Model file for the job. Use its own axes, mm. Face numbers are marked on the shaded views. A direction names the side the tool comes from. Round coordinates to 2 decimals unless told otherwise and drop trailing zeros. Order: outer loops, then holes, each group sorted by start corner. A loop starts at its lowest first (then second) coordinate and runs counter-clockwise, first axis right, second up. Notation, with made-up numbers: (40.25, 46) - (70.25, 46) arc R4 ccw to (70.25, 52) - close; hole circle Ø4 at (-9.5, 58.25). An arc over 180 degrees is marked (long way). Use one line per item in the form item = value.
from build123d import *

# Parameters (mm, degrees)
SKETCH1_W           = 40
SKETCH1_H           = 20
BOSS_EXTRUDE1_DEPTH = 10
SKETCH2_R           = 5.15
CUT_EXTRUDE1_DEPTH  = 2.4
CUT_EXTRUDE2_DEPTH  = 31
FILLET1_R           = 2
SKETCH4_W           = 0.5
SKETCH4_H           = 10
CUT_EXTRUDE3_DEPTH  = 0.5
SKETCH5_W           = 0.5
SKETCH5_H           = 20
CUT_EXTRUDE4_DEPTH  = 0.5
SKETCH6_W           = 0.5
SKETCH6_H           = 10
CUT_EXTRUDE5_DEPTH  = 0.5
FILLET2_R           = 1
SKETCH8_W           = 14.3
SKETCH8_H           = 7
CUT_EXTRUDE7_DEPTH  = 3.3
SKETCH9_R           = 1.6
CUT_EXTRUDE8_DEPTH  = 10
CUT_EXTRUDE9_DEPTH  = 1.25
FILLET4_R           = 0.5


# Some blends are built 0.0001 mm under size
with BuildPart() as part:
    # Sketch1 → Boss-Extrude1 (new body)
    with BuildSketch(Plane(origin=(0, 0, 0), x_dir=(1, 0, 0), z_dir=(0, 1, 0))):
        Rectangle(SKETCH1_W, SKETCH1_H)
    extrude(amount=BOSS_EXTRUDE1_DEPTH)

    # Sketch2 → Cut-Extrude1 (cut)
    with BuildSketch(Plane.XZ):
        with Locations(Location((0, 0, 0), (0, 0, 270))):
            Circle(SKETCH2_R)
        with Locations(Location((12, 0, 0), (0, 0, 270))):
            Circle(SKETCH2_R)
        with Locations(Location((-12, 0, 0), (0, 0, 270))):
            Circle(SKETCH2_R)
    extrude(amount=-CUT_EXTRUDE1_DEPTH, mode=Mode.SUBTRACT)

    # Sketch3 → Cut-Extrude2 (cut, through all)
    with BuildSketch(Plane.XY.offset(10)):
        Polygon((18, 10), (14.75, 6.75), (14.75, 5.25), (13.25, 5.25), (13.25, 6.75), (10, 10), align=None)
    extrude(amount=-CUT_EXTRUDE2_DEPTH, mode=Mode.SUBTRACT)

    # Fillet1
    fillet1_edges = [part.edges().sort_by_distance(p)[0] for p in [
        (20, 10, 0),
        (-20, 10, 0),
        (-20, 5, -10),
        (20, 5, -10),
        (20, 5, 10),
        (-20, 5, 10),
    ]]
    fillet(fillet1_edges, radius=FILLET1_R - 0.0001)  # a hair under: the kernel refuses the full size

    # Sketch4 → Cut-Extrude3 (cut)
    with BuildSketch(Plane.XY.offset(10)):
        with Locations((0, 5)):
            Rectangle(SKETCH4_W, SKETCH4_H)
    extrude(amount=-CUT_EXTRUDE3_DEPTH, mode=Mode.SUBTRACT)

    # Sketch5 → Cut-Extrude4 (cut)
    with BuildSketch(Plane(origin=(0, 10, 0), x_dir=(1, 0, 0), z_dir=(0, 1, 0))):
        Rectangle(SKETCH5_W, SKETCH5_H)
    extrude(amount=-CUT_EXTRUDE4_DEPTH, mode=Mode.SUBTRACT)

    # Sketch6 → Cut-Extrude5 (cut)
    with BuildSketch(Plane(origin=(0, 0, -10), x_dir=(-1, 0, 0), z_dir=(0, 0, -1))):
        with Locations((0, 5)):
            Rectangle(SKETCH6_W, SKETCH6_H)
    extrude(amount=-CUT_EXTRUDE5_DEPTH, mode=Mode.SUBTRACT)

    # Fillet2
    # the kernel refuses this fillet: 1 mm, written as the material it takes off along each edge
    with BuildSketch(Plane(origin=(10, 10, 11.035533906), x_dir=(0.7071067811865476, -0.7071067811865476, 0), z_dir=(0, 0, -1))) as fillet2_piece_1:
        with BuildLine():
            CenterArc((FILLET2_R * 0.414213562373, FILLET2_R), FILLET2_R, 225, 45)
            Line((-FILLET2_R * 0.292893218813, FILLET2_R * 0.292893218813), (0, 0))
            Line((0, 0), (FILLET2_R * 0.414213562373, 0))
        make_face()
    extrude(amount=22.071067812, mode=Mode.SUBTRACT)
    with BuildSketch(Plane(origin=(18, 10, 11.781961717), x_dir=(-0.7071067811865406, -0.7071067811865547, 0), z_dir=(0, 0, -1))) as fillet2_piece_2:
        with BuildLine():
            CenterArc((0.504002289, -1), FILLET2_R, 90, 65.527591719)
            Line((-0.406158578, -0.585745012), (-0.497174665, -0.544319513))
            ThreePointArc((-0.497174665, -0.544319513), (-0.070781389, 0.070639967), (-0.070710678, 0.070710678))
            Line((-0.070710678, 0.070710678), (0, 0.1))
            Line((0, 0.1), (0.504002289, 0.1))
            Line((0.504002289, 0.1), (0.504002289, 0))
        make_face()
    extrude(amount=23.563923435, mode=Mode.SUBTRACT)

    # Sketch8 → Cut-Extrude7 (cut, symmetric)
    with BuildSketch(Plane.XY):
        with Locations((0, 6.5)):
            Rectangle(SKETCH8_W, SKETCH8_H)
    extrude(amount=CUT_EXTRUDE7_DEPTH, both=True, mode=Mode.SUBTRACT)

    # Sketch9 → Cut-Extrude8 (cut)
    with BuildSketch(Plane.XY.offset(10)):
        with Locations((0, 6.5)):
            Circle(SKETCH9_R)
    extrude(amount=-CUT_EXTRUDE8_DEPTH, mode=Mode.SUBTRACT)

    # Sketch10 → Cut-Extrude9 (cut, symmetric)
    with BuildSketch(Plane.XY.offset(7)):
        Polygon((-2.76, 8.093486743), (-2.76, 10), (2.76, 10), (2.76, 8.081939738), (2.76, 4.906513257), (0, 3.313026514), (-2.76, 4.906513257), align=None)
    extrude(amount=CUT_EXTRUDE9_DEPTH, both=True, mode=Mode.SUBTRACT)

    # Fillet4
    fillet4_edges = [part.edges().sort_by_distance(p)[0] for p in [
        (3.7, 10, -3.3),
        (7.15, 10, 0),
        (3.7, 10, 3.3),
        (-3.7, 10, 3.3),
        (-7.15, 10, 0),
        (-3.7, 10, -3.3),
    ]]
    fillet(fillet4_edges, radius=FILLET4_R)


solid = part.part
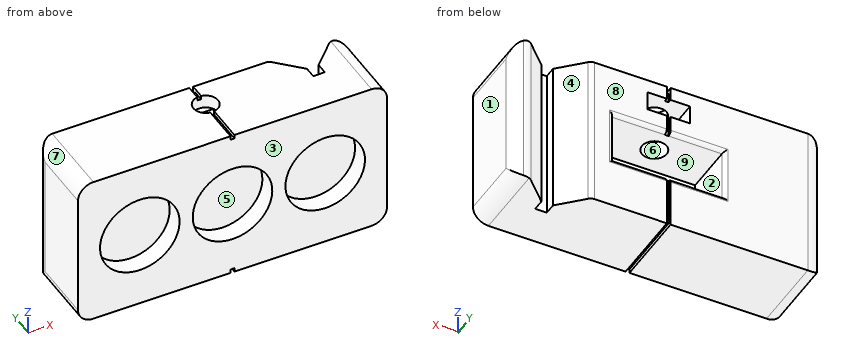
(1) Slice it at B-B on z = -6. Give the cut face in (x, y), then the cut area to 3 significant figures.
Report:
outline = (-20, 0) - (20, 0) - (20, 8) arc R2 ccw to (18.7, 9.87) arc R1 ccw to (17.64, 9.64) - (14.75, 6.75) - (14.75, 5.25) - (13.25, 5.25) - (13.25, 6.75) - (10.29, 9.71) arc R1 ccw to (9.59, 10) - (0.25, 10) - (0.25, 9.5) - (-0.25, 9.5) - (-0.25, 10) - (-18, 10) arc R2 ccw to (-20, 8) - close
area = 380 mm2
(2) Slice it at A-A on y = 2. Give the cut face in (x, z).
Report:
outline = (-20, -8) arc R2 ccw to (-18, -10) - (-0.25, -10) - (-0.25, -9.5) - (0.25, -9.5) - (0.25, -10) - (18, -10) arc R2 ccw to (20, -8) - (20, 8) arc R2 ccw to (18, 10) - (0.25, 10) - (0.25, 9.5) - (-0.25, 9.5) - (-0.25, 10) - (-18, 10) arc R2 ccw to (-20, 8) - close; hole circle Ø10.3 at (-12, 0); hole circle Ø10.3 at (0, 0); hole circle Ø10.3 at (12, 0)
(3) Pin check, flat tips, straight feed: pin 1 (2 mm diameter, centred on x = -3, z = 0.5, fed in from +Y); pin 2 (1.6 mm diameter, centred on x = 13.5, z = -1.5, fed in from +Y); pin 3 (1.9 mm diameter, centred on y = 9, z = 9.5, fed in from -X). Stop position of each tip, or through.
Report:
pin_1 = 3
pin_2 = 7.3
pin_3 = -19.9
(4) Tool access for the marked faces 5, 6, 7, 8 and 9: list every direction of +Z, -Z, +X, -X, +Y, -Y with a clear straight run to the whole face (end or side of a thin tool).
Report:
face_5 = -Y
face_6 = +Z
face_7 = +Z, -X, +Y, -Y
face_8 = +Z, -Z, +X, -X, +Y
face_9 = +Y
(5) Slice it at C-C on x = -12. Give the cut face in (y, z), then the cut area to 3 significant figures.
Report:
outline = (0, -10) - (10, -10) - (10, 10) - (0, 10) - (0, 5.15) - (2.4, 5.15) - (2.4, -5.15) - (0, -5.15) - close
area = 175 mm2
(6) Pull direction X, two halves, no side cores. Call the marked faces 1, 2, 3 and 4: released by +X, released by -X, zero draft, split by the parting line, or undercut.
Report:
face_1 = released by +X
face_2 = undercut
face_3 = zero draft
face_4 = undercut
(7) Probe probe 1 along X at (y, z) = (0.7, 0); probe 2 along Z at (x, y) = (2.5, 5.5); probe 3 along Z at (x, y) = (3.5, 4.5). List the from-to ranges inside material, lowest first. Write a range as [from, to].
Report:
probe_1 = [-20, -17.15], [-6.85, -5.15], [5.15, 6.85], [17.15, 20]
probe_2 = [-10, -3.3], [3.3, 5.75], [8.25, 10]
probe_3 = [-10, -3.3], [3.3, 10]
